Build history of the part. All positions in model axes, mm. Face numbers are marked on the shaded views. A direction names the side the tool comes from. Give positions to 0.01 mm unless a question says otherwise; leave off trailing zeros. Order: outer loops, then holes, each group sorted by start corner. A loop starts at its lowest first (then second) coordinate and runs counter-clockwise, first axis right, second up. Notation, with made-up numbers: M 56,53.25 L 87,53.25 A16 cw 87,73.25 Z; hole C -23,87.25 d1. An arc over 180 degrees is marked long. Answer as CSV lines item,"result".
from build123d import *

# Parameters (mm, degrees)
ESQUISSE1_W             = 8
ESQUISSE1_H             = 3.75
ENL_V_MAT_EXTRU_2_DEPTH = 25


with BuildPart() as part:
    # Esquisse1 → R_volution1 (revolve)
    with BuildSketch(Plane.XY, mode=Mode.PRIVATE) as r_volution1_sk:
        with Locations((-8.673814, 5.625)):
            Rectangle(ESQUISSE1_W, ESQUISSE1_H)
    revolve(r_volution1_sk.sketch.rotate(Axis((-26.499793814, 0, 0), (1, 0, 0)), 90), axis=Axis((-26.499793814, 0, 0), (1, 0, 0)))  # turned: the seam where the file's is

    # Esquisse2 → Enl_v. mat.-Extru.2 (cut, symmetric)
    with BuildSketch(Plane.XY):
        with BuildLine():
            Line((-8.673814, 0), (-4.141062675, 0))
            Line((-4.141062675, 0), (-4.145756794, 1))
            Line((-4.145756794, 1), (-7.673814, 1))
            ThreePointArc((-7.673814, 1), (-8.380920781, 0.707106781), (-8.673814, 0))
        make_face()
        with BuildLine():
            Line((-7.673814, -1), (-4.136368556, -1))
            Line((-4.136368556, -1), (-4.141062675, 0))
            Line((-4.141062675, 0), (-8.673814, 0))
            ThreePointArc((-8.673814, 0), (-8.380920781, -0.707106781), (-7.673814, -1))
        make_face()
    extrude(amount=ENL_V_MAT_EXTRU_2_DEPTH, both=True, mode=Mode.SUBTRACT)


solid = part.part
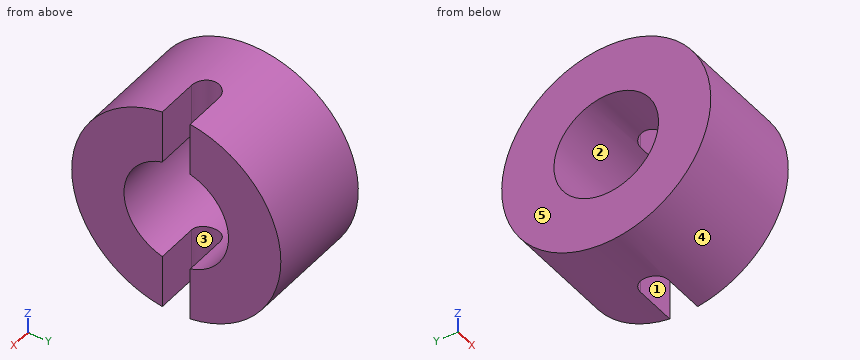
Item 1: Drop flat-ended pins along their axis: pin 1 (3 mm diameter, centred on x = -11, z = 4.5, fed in from +Y); pin 2 (4 mm diameter, centred on x = -5.5, z = -4, fed in from +Y); pin 3 (3.5 mm diameter, centred on x = -5.5, z = 5, fed in from -Y). Give the stop position or say it passes through.
Geometry says:
pin 1,"stops at y = 6.87"
pin 2,"stops at y = 7.23"
pin 3,"stops at y = -6.76"
Item 2: Probe line 1 along Y through (x, z) = (-7.5, 0); line 2 along Z through (x, y) = (-11, 1); line 3 along Y through (x, z) = (-10.25, -1.5). List the from-to ranges inside material, lowest first. Write a range as from..to.
Geometry says:
line 1,"y = -7.5..-3.75, 3.75..7.5"
line 2,"z = -7.43..-3.61, 3.61..7.43"
line 3,"y = -7.35..-3.44, 3.44..7.35"
Item 3: Pull direction Y, two halves, no side cores. Call the marked faces 3, 4 and 5: released by +Y, released by -Y, zero draft, split by the parting line, or undercut.
Geometry says:
face 3,"undercut"
face 4,"split by the parting line"
face 5,"zero draft"
Item 4: Band-saw the part on C-C (x = -10.5). Give the cut face in (y, z).
Geometry says:
outline,"C 0,0 d15; hole C 0,0 d7.5"
Item 5: Band-saw the part on A-A (y = 0). Give the cut face in (x, z), and give its area (3 significant figures).
Geometry says:
outline,"M -12.67,-7.5 L -8.67,-7.5 L -8.67,-3.75 L -12.67,-3.75 Z; M -12.67,3.75 L -8.67,3.75 L -8.67,7.5 L -12.67,7.5 Z"
area,"30.0 mm2"
Item 6: Band-saw the part on D-D (z = 4.5). Give the cut face in (x, y).
Geometry says:
outline,"M -12.67,-6 L -4.67,-6 L -4.67,-1 L -7.67,-1 A1 cw -7.67,1 L -4.67,1 L -4.67,6 L -12.67,6 Z"
Item 7: 3-axis set-ups, long thin cutter, end or side, ignore diameter. For the marked faces 1 and 2: which of +Z, -Z, +X, -X, +Y, -Y reach the whole face in a straight line?
Geometry says:
face 1,"+Z, -Z, +X"
face 2,"+X, -X"
Item 8: Band-saw the part on B-B (z = 0). Give the cut face in (x, y).
Geometry says:
outline,"M -12.67,-7.5 L -4.67,-7.5 L -4.67,-3.75 L -12.67,-3.75 Z; M -12.67,3.75 L -4.67,3.75 L -4.67,7.5 L -12.67,7.5 Z"
